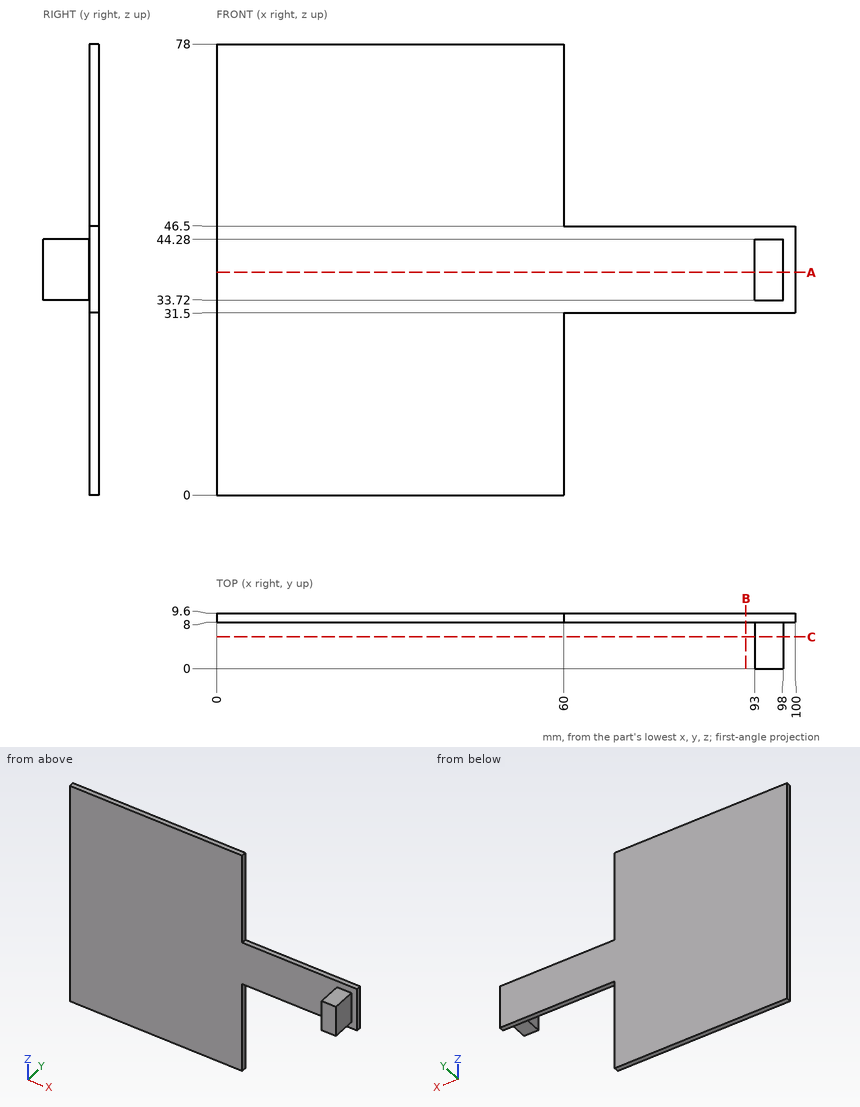
Geometry: see drawing. Coordinates: mm, zero at the bounding-box minimum. Give positions to 0.01 mm unless a question says otherwise; leave off trailing zeros. Order: outer loops, then holes, each group sorted by start corner. A loop starts at its lowest first (then second) coordinate and runs counter-clockwise, first axis right, second up.
Q1. Contact query for flat-ended pins moving along their axis: pin 1 Ø5.5 at (x, y) = (96, 4) entering from +Z; pin 2 Ø8 at (x, z) = (17.5, 42.5) entering from -Y; pin 3 Ø0.5 at (y, z) = (9, 11) entering from +X. Output: stop coordinate, or through.
Checked values:
pin 1: stops at z = 44.28
pin 2: stops at y = 8
pin 3: stops at x = 60
Q2. Ray query, probe 1 along X at (y, z) = (8.25, 50.5); probe 2 along Y at (x, z) = (24, 46.5); probe 3 along X at (y, z) = (7.75, 37.5). Return the intervals inside material, ascending.
Checked values:
probe 1: x = 0 to 60
probe 2: y = 8 to 9.6
probe 3: x = 93 to 98
Q3. Section B-B on x = 91.5. Output: boundary loops of the cut face in (y, z), and give its area (3 significant figures).
Checked values:
outline: (8, 31.5) - (9.6, 31.5) - (9.6, 46.5) - (8, 46.5) - close
area: 24.0 mm2
Q4. Section C-C on y = 5.5. Output: boundary loops of the cut face in (x, z), and give its area (3 significant figures).
Checked values:
outline: (93, 33.72) - (98, 33.72) - (98, 44.28) - (93, 44.28) - close
area: 52.8 mm2
Q5. Section A-A on z = 38.5. Output: boundary loops of the cut face in (x, y).
Checked values:
outline: (0, 8) - (93, 8) - (93, 0) - (98, 0) - (98, 8) - (100, 8) - (100, 9.6) - (0, 9.6) - close
